Autodesk Inventor part; units mm, degrees
ref_plane "YZ Plane" through (0, 0, 0) normal (1, 0, 0) x (0, 1, 0)
ref_plane "XZ Plane" through (0, 0, 0) normal (0, 1, 0) x (-1, 0, 0)
ref_plane "XY Plane" through (0, 0, 0) normal (0, 0, 1) x (1, 0, 0)
sketch "Skizze6" plane through (0, 0, 0) normal (0, 0, 1) x (1, 0, 0)
  line L0 (0, 0) -> (-20, 0)
  line L1 (-20, 0) -> (-20, 24)
  line L2 (-20, 24) -> (0, 24)
  line L3 (0, 24) -> (0, 0)
  circle A0 centre (-5, 21) radius 1.65
  circle A1 centre (-5, 14.5) radius 1.65
  dimension "d29" = 20
  dimension "d30" = 24
  dimension "d31" = 3.3
  dimension "d32" = 3.3
  dimension "d33" = 3
  dimension "d34" = 6.5
  dimension "d35" = 5
extrude "Extrusion5" add sketch "Skizze6" along normal blind 14
sketch "Skizze7" plane through (-20, 0, 0) normal (0, -1, 0) x (1, 0, 0)
  line L0 (0, 0) -> (20, 0)
  line L1 (20, 0) -> (20, 14)
  line L2 (0, 14) -> (20, 14)
  line L3 (0, 0) -> (0, 14)
  circle A0 centre (10, 7) radius 4
  dimension "d38" = 8
  dimension "d39" = 10
extrude "Extrusion6" cut sketch "Skizze7" against normal through all contours A0
sketch "Skizze8" plane through (0, 0, 14) normal (0, 0, 1) x (1, 0, 0)
  line L0 (0, 24) -> (-20, 24)
  line L1 (-20, 24) -> (-20, 0)
  line L2 (-20, 0) -> (0, 0)
  line L3 (0, 0) -> (0, 24)
  circle A0 centre (-5, 14.5) radius 1.65
  circle A1 centre (-5, 21) radius 1.65
  line L4 (-5, 14.5) -> (-5, 31.6413) construction
  line L5 (-1.75, 14.5) -> (-1.75, 31.6413)
  line L6 (-8.25, 31.6413) -> (-8.25, 14.5)
  arc A2 (-8.25, 14.5) -> (-1.75, 14.5) centre (-5, 14.5) ccw
  arc A3 (-1.75, 31.6413) -> (-8.25, 31.6413) centre (-5, 31.6413) ccw
  point P0 (-5, 23.0707)
  dimension "d42" = 6.5
extrude "Extrusion7" cut sketch "Skizze8" against normal blind 3 contours L5 A2 L6 L0 | L0 L6 A3 L5 | A0 | A1
sketch "Skizze9" plane through (-20, 0, 0) normal (0, -1, 0) x (1, 0, 0)
  circle A0 centre (10, 7) radius 4
  line L0 (0, 0) -> (20, 0)
  line L1 (20, 0) -> (20, 14)
  line L2 (0, 14) -> (20, 14)
  line L3 (0, 0) -> (0, 14)
  circle A1 centre (10, 7) radius 7.25
  line L4 (20, 17) -> (0, 17)
  line L5 (0, 17) -> (0, -3)
  line L6 (0, -3) -> (20, -3)
  line L7 (20, -3) -> (20, 17)
  line L8 (20, 17) -> (0, -3) construction
  line L9 (0, 17) -> (20, -3) construction
  line L10 (0, 17) -> (20, 17)
  line L11 (20, 17) -> (20, 20)
  line L12 (20, 20) -> (0, 20)
  line L13 (0, 20) -> (0, 17)
  dimension "d45" = 14.5
  dimension "d46" = 20
  dimension "d47" = 20
  dimension "d50" = 3
extrude "Extrusion8" add sketch "Skizze9" along normal blind 15 contours L3 L2 A1 L0 | L0 A1 L7 L6 L5 | L5 L4 L7 L2 A1 | A1 L2 L1 L0 | L13 L12 L11 L4
sketch "Skizze10" plane through (-20, 24, 0) normal (-1, 0, 0) x (0, 0, 1)
  line L0 (14.25, -39) -> (14.25, -24)
  circle A0 centre (15.3846, -32.1377) radius 1.4
  point P0 (0, -24)
  dimension "d51" = 2.8
hole "Bohrung2" at (-20, -8.1377, 15.3846) direction (1, 0, 0) diameter 2.8 end through all counterbore diameter 6.5 counterbore depth 4
properties part number "40_XYZstage_micrometer_motorized_nema8_nanotec_adapter_z"
Geometry check sheet. Reference: the model listing, model coordinates, mm. A direction names the side the tool comes from. Give positions to 0.01 mm unless a question says otherwise; leave off trailing zeros. Loops run counter-clockwise (first coordinate to the right, second up) from the corner with the lowest first, then second, coordinate; pieces in that order, holes last. Notation, with made-up numbers: (26, -39.75) - (80, -39.75) arc R25 ccw to (80, -3.75) - close; hole circle Ø2 at (66.5, -24). An arc over 180 degrees is marked (long way). Use CSV: the item, a comma, the result in double quotes. Start each with the question number.
Q1. Section check C-C, the plane z = 5.25. Record the cut outline in (x, y).
Q2. Section check B-B, the plane y = 14. Record the cut outline in (x, z).
Q3. Go/stop test with flat-tipped pins: pin 1 Ø7 at (x, z) = (-10, 7) entering from +Y; pin 2 Ø4 at (x, z) = (-6.5, 6.5) entering from -Y; pin 3 Ø6 at (x, y) = (-12.5, 6.5) entering from +Z; pin 4 Ø3 at (x, z) = (-6.5, 16.5) entering from +Y. Record where each tip stops, or that it passes through.
Q4. Scan lines: probe 1 along Y at (x, z) = (-5, 4); probe 2 along Z at (x, y) = (-10, -4); probe 3 along Y at (x, z) = (-6, 2.75). Record each from-to range of solid material in increasing order. Write a range as from..to.
Q5. Access from +Z, -Z, +X, -X, +Y, -Y to the whole of each face (thin tool, end or side, straight path). Record for faces 1 (the face through (-10, 0, 17)), 2 (the face through (-10, 12, 0)), 3 (the face through (-17.97, -11.36, 14.96)), 4 (the face through (-6.65, -7.4, 13.43)), 5 (the face through (-1.75, 19, 13)).
Q6. Section check A-A, the plane x = -5. Record the cut outline in (y, z).
Q7. Section check D-D, the plane x = -14.75. Record the cut outline in (y, z), and give its area (3 significant figures).
Q8. Release check for a two-part mould opening along Y. For faces 6 (the face through (-10, 12, 14)), 7 (the face through (-10, 0, -1)), 8 (the face through (-16, -6.7, 16.1)), 9 (the face through (-3.426, 20.504, 5.423)) record: +Y half, -Y half, draft (parallel to the pull), parting line (faces both ways), or undercut.
Findings below:
1,outline,"(-20, -15) - (-17.04, -15) - (-17.04, 0) - (-13.6, 0) - (-13.6, 24) - (-20, 24) - close; (-6.4, 0) - (-2.96, 0) - (-2.96, -15) - (0, -15) - (0, 24) - (-6.4, 24) - (-6.4, 21.87) arc R1.65 cw (long way) to (-6.4, 20.13) - (-6.4, 15.37) arc R1.65 cw (long way) to (-6.4, 13.63) - close"
2,outline,"(-20, 0) - (-6.57, 0) - (-6.57, 4.94) arc R4 cw (long way) to (-6.57, 9.06) - (-6.57, 11) - (-8.21, 11) - (-8.21, 14) - (-20, 14) - close; (-3.43, 0) - (0, 0) - (0, 14) - (-1.79, 14) - (-1.79, 11) - (-3.43, 11) - close"
3,pin 1,"passes through"
3,pin 2,"stops at y = 0"
3,pin 3,"stops at z = 14"
3,pin 4,"stops at y = 0"
4,probe 1,"y = 0..12.85, 16.15..19.35, 22.65..24"
4,probe 2,"z = -3..-0.25, 14.25..20"
4,probe 3,"y = 0..13.19, 15.81..19.69, 22.31..24"
5,face 1,"+Z, +X, -X, +Y"
5,face 2,"-Z, +X, -X, +Y"
5,face 3,"-X"
5,face 4,"-Y"
5,face 5,"+Z, +Y"
6,outline,"(-15, -3) - (0, -3) - (0, 0) - (12.85, 0) - (12.85, 11) - (11.25, 11) - (11.25, 14) - (0, 14) - (0, 20) - (-15, 20) - (-15, 12.25) - (0, 12.25) - (0, 1.75) - (-15, 1.75) - close; (16.15, 0) - (19.35, 0) - (19.35, 11) - (16.15, 11) - close; (22.65, 0) - (24, 0) - (24, 11) - (22.65, 11) - close; hole circle Ø2.8 at (-8.14, 15.38)"
7,outline,"(-15, -3) - (0, -3) - (0, 0) - (24, 0) - (24, 14) - (0, 14) - (0, 20) - (-15, 20) - (-15, 12.48) - (0, 12.48) - (0, 1.52) - (-15, 1.52) - close; hole circle Ø2.8 at (-8.14, 15.38)"
7,area,"511 mm^2"
8,face 6,"draft"
8,face 7,"+Y half"
8,face 8,"undercut"
8,face 9,"undercut"
